from build123d import *

# Parameters (mm, degrees)
F0_W           = 60
F0_H           = 35
F1_DEPTH       = 4
F3_DEPTH       = 3
F4_R           = 5.08
F5_W           = 27
F5_H           = 19
F6_DEPTH       = 25.4
F8_D           = 3.5
F8_CSINK_D     = 6
F8_CSINK_ANGLE = 90
F9_D           = 3
F10_T1_DEPTH   = 58
F10_T3_DEPTH   = 33
F10_T5_DEPTH   = 5.5
F10_S9_W       = 1
F10_S9_H       = 1
F10_T10_DEPTH  = 1
F10_S15_W      = 1
F10_S15_H      = 1
F10_T16_DEPTH  = 1
F10_S21_W      = 1
F10_S21_H      = 1
F10_T22_DEPTH  = 1
F10_S27_W      = 1
F10_S27_H      = 1
F10_T28_DEPTH  = 1


# Not quite as in the source:
# - a fillet or chamfer that OpenCascade refuses, or shapes differently, is made with other operations: its cross-section is extruded or revolved along the edge and cut away or added


with BuildPart() as f1:
    # F0 (on Top) → F1 (new body)
    with BuildSketch(Plane.XY):
        Rectangle(F0_W, F0_H)
    extrude(amount=F1_DEPTH)

    # F2 (on face) → F3 (cut)
    with BuildSketch(Plane.XY.offset(4)):
        Polygon((-27.3, 0), (-12.5, -11.5), (12.5, -11.5), (27.3, 0), (12.5, 11.5), (-12.5, 11.5), align=None)
    extrude(amount=-F3_DEPTH, mode=Mode.SUBTRACT)

    # F4
    f4_edges = [f1.edges().sort_by_distance(p)[0] for p in [
        (12.5, 11.5, 2.5),
        (12.5, -11.5, 2.5),
        (-12.5, -11.5, 2.5),
        (-12.5, 11.5, 2.5),
        (27.3, 0, 2.5),
        (-27.3, 0, 2.5),
    ]]
    fillet(f4_edges, radius=F4_R)

    # F5 (on face) → F6 (cut)
    with BuildSketch(Plane.XY.offset(1)):
        Rectangle(F5_W, F5_H)
    extrude(amount=-F6_DEPTH, mode=Mode.SUBTRACT)

    # F8 (through all)
    with Locations(Plane.XY.offset(4)):
        with Locations((-26, 13.5), (26, 13.5), (26, -13.5), (-26, -13.5)):
            CounterSinkHole(F8_D / 2, F8_CSINK_D / 2, counter_sink_angle=F8_CSINK_ANGLE)

    # F9 (through all)
    with Locations(Plane.XY.offset(4)):
        with Locations((-20.3, 0), (20.3, 0)):
            Hole(F9_D / 2)

    # F10: fillet of radius 1 on 8 edges, made by hand

    # F10_s2 → F10_t1 (cut)
    with BuildSketch(Plane.YZ.offset(-29)):
        with BuildLine():
            ThreePointArc((16.5, 4), (17.2071067812, 3.7071067812), (17.5, 3))
            Line((17.5, 3), (17.5, 4))
            Line((17.5, 4), (16.5, 4))
        make_face()
        with BuildLine():
            ThreePointArc((-16.5, 4), (-17.2071067812, 3.7071067812), (-17.5, 3))
            Line((-17.5, 3), (-17.5, 4))
            Line((-17.5, 4), (-16.5, 4))
        make_face()
    extrude(amount=F10_T1_DEPTH, mode=Mode.SUBTRACT)

    # F10_s4 → F10_t3 (cut)
    with BuildSketch(Plane.XZ.offset(-16.5)):
        with BuildLine():
            ThreePointArc((-29, 4), (-29.7071067812, 3.7071067812), (-30, 3))
            Line((-30, 3), (-30, 4))
            Line((-30, 4), (-29, 4))
        make_face()
        with BuildLine():
            ThreePointArc((29, 4), (29.7071067812, 3.7071067812), (30, 3))
            Line((30, 3), (30, 4))
            Line((30, 4), (29, 4))
        make_face()
    extrude(amount=F10_T3_DEPTH, mode=Mode.SUBTRACT)

    # F10_s6 → F10_t5 (cut)
    with BuildSketch(Plane.XY.offset(-2.5)):
        with BuildLine():
            ThreePointArc((30, -16.5), (29.7071067812, -17.2071067812), (29, -17.5))
            Line((29, -17.5), (30, -17.5))
            Line((30, -17.5), (30, -16.5))
        make_face()
        with BuildLine():
            ThreePointArc((29, 17.5), (29.7071067812, 17.2071067812), (30, 16.5))
            Line((30, 16.5), (30, 17.5))
            Line((30, 17.5), (29, 17.5))
        make_face()
        with BuildLine():
            ThreePointArc((-30, -16.5), (-29.7071067812, -17.2071067812), (-29, -17.5))
            Line((-29, -17.5), (-30, -17.5))
            Line((-30, -17.5), (-30, -16.5))
        make_face()
        with BuildLine():
            ThreePointArc((-29, 17.5), (-29.7071067812, 17.2071067812), (-30, 16.5))
            Line((-30, 16.5), (-30, 17.5))
            Line((-30, 17.5), (-29, 17.5))
        make_face()
    extrude(amount=F10_T5_DEPTH, mode=Mode.SUBTRACT)


with BuildPart() as f10_tool8:
    # F10_s9 → F10_t10 (new body)
    with BuildSketch(Plane.XY.offset(3)):
        with Locations((29.5, 17)):
            Rectangle(F10_S9_W, F10_S9_H)
    extrude(amount=F10_T10_DEPTH)

    # F10_s11 → F10_t12 (revolve, cut)
    with BuildSketch(Plane(origin=(29, 16.5, 3), x_dir=(-0.7071067812, -0.7071067812, 0), z_dir=(-0.7071067812, 0.7071067812, 0))):
        with BuildLine():
            ThreePointArc((0, -1), (1, 0), (0, 1))
            Line((0, 1), (0, -1))
        make_face()
    revolve(axis=Axis((29, 16.5, 3), (0, 0, 1)), mode=Mode.SUBTRACT)


with BuildPart() as f1_1:
    add(f1.part)

    # F10_t7: cut F10_tool8
    add(f10_tool8.part, mode=Mode.SUBTRACT)


with BuildPart() as f10_tool14:
    # F10_s15 → F10_t16 (new body)
    with BuildSketch(Plane.XY.offset(3)):
        with Locations((-29.5, 17)):
            Rectangle(F10_S15_W, F10_S15_H)
    extrude(amount=F10_T16_DEPTH)

    # F10_s17 → F10_t18 (revolve, cut)
    with BuildSketch(Plane(origin=(-29, 16.5, 3), x_dir=(0.7071067812, -0.7071067812, 0), z_dir=(-0.7071067812, -0.7071067812, 0))):
        with BuildLine():
            ThreePointArc((0, -1), (1, 0), (0, 1))
            Line((0, 1), (0, -1))
        make_face()
    revolve(axis=Axis((-29, 16.5, 3), (0, 0, 1)), mode=Mode.SUBTRACT)


with BuildPart() as f1_2:
    add(f1_1.part)

    # F10_t13: cut F10_tool14
    add(f10_tool14.part, mode=Mode.SUBTRACT)


with BuildPart() as f10_tool20:
    # F10_s21 → F10_t22 (new body)
    with BuildSketch(Plane.XY.offset(3)):
        with Locations((-29.5, -17)):
            Rectangle(F10_S21_W, F10_S21_H)
    extrude(amount=F10_T22_DEPTH)

    # F10_s23 → F10_t24 (revolve, cut)
    with BuildSketch(Plane(origin=(-29, -16.5, 3), x_dir=(0.7071067812, 0.7071067812, 0), z_dir=(0.7071067812, -0.7071067812, 0))):
        with BuildLine():
            ThreePointArc((0, -1), (1, 0), (0, 1))
            Line((0, 1), (0, -1))
        make_face()
    revolve(axis=Axis((-29, -16.5, 3), (0, 0, 1)), mode=Mode.SUBTRACT)


with BuildPart() as f1_3:
    add(f1_2.part)

    # F10_t19: cut F10_tool20
    add(f10_tool20.part, mode=Mode.SUBTRACT)


with BuildPart() as f10_tool26:
    # F10_s27 → F10_t28 (new body)
    with BuildSketch(Plane.XY.offset(3)):
        with Locations((29.5, -17)):
            Rectangle(F10_S27_W, F10_S27_H)
    extrude(amount=F10_T28_DEPTH)

    # F10_s29 → F10_t30 (revolve, cut)
    with BuildSketch(Plane(origin=(29, -16.5, 3), x_dir=(-0.7071067812, 0.7071067812, 0), z_dir=(0.7071067812, 0.7071067812, 0))):
        with BuildLine():
            ThreePointArc((0, -1), (1, 0), (0, 1))
            Line((0, 1), (0, -1))
        make_face()
    revolve(axis=Axis((29, -16.5, 3), (0, 0, 1)), mode=Mode.SUBTRACT)


with BuildPart() as f1_4:
    add(f1_3.part)

    # F10_t25: cut F10_tool26
    add(f10_tool26.part, mode=Mode.SUBTRACT)


solid = f1_4.part
Verification items for the finished model (mm, model axes). A direction names the side the tool comes from. Round coordinates to 2 decimals unless told otherwise and drop trailing zeros. Loops run counter-clockwise (first coordinate to the right, second up) from the corner with the lowest first, then second, coordinate; pieces in that order, holes last. Notation, with made-up numbers: (7.25, -22) - (13.25, -22) arc R29 ccw to (13.25, -1) - close; hole circle Ø7 at (87, 30). An arc over 180 degrees is marked (long way). Answer in a Markdown table with one row per item. Add a question column.
Q1. Release check for a two-part mould opening along Y. For faces 1 (the face through (0, 17.5, 1)), 2 (the face through (0, 15, 4)), 3 (the face through (2, 10, 1)) record: pulls with the +Y half, pulls with the -Y half, needs draft (parallel to the pull), parting line crosses it, or undercut.
Q2. Section check B-B on y = 0. Enter the section's corners in (x, z), plus the area to 3 significant figures.
Q3. Material ranges on line 1 (Y direction, x = 26, z = 1.65); line 2 (Y direction, x = 2, z = 1.8); line 3 (Y direction, x = -3.5, z = 0.8), recorded low to high.
Q4. Tool access check on faces 4 (the face through (18.06, 7.18, 2.52)), 5 (the face through (21.8, 0.07, 0.49)). Record the directions out of +Z, -Z, +X, -X, +Y, -Y that give a thin tool (end or side, any length) a straight path to the whole face; none if there is none.
Q5. Section check A-A on z = 1.85. Enter the section's corners in (x, y), plus the area to 3 significant figures.
Q6. Section check C-C on x = -20.3. Enter the section's corners in (y, z).
Q7. Gauge pin test, flat end, axial feed: pin 1 (12 mm diameter, centred on x = -10.5, y = -2.5, fed in from +Z). Record the tip position at first contact, or that the pin passes through.
Found:
| question | item | result |
|---|---|---|
| 1 | face 1 | pulls with the +Y half |
| 1 | face 2 | needs draft |
| 1 | face 3 | undercut |
| 2 | outline | (-30, 0) - (-21.8, 0) - (-21.8, 1) - (-24.1, 1) - (-24.1, 4) - (-29, 4) arc R1 ccw to (-30, 3) - close; (-18.8, 0) - (-13.5, 0) - (-13.5, 1) - (-18.8, 1) - close; (13.5, 0) - (18.8, 0) - (18.8, 1) - (13.5, 1) - close; (21.8, 0) - (30, 0) - (30, 3) arc R1 ccw to (29, 4) - (24.1, 4) - (24.1, 1) - (21.8, 1) - close |
| 2 | area | 62.0 mm² |
| 3 | line 1 | y = -17.5 to -15.25, -11.75 to 11.75, 15.25 to 17.5 |
| 3 | line 2 | y = -17.5 to -11.5, 11.5 to 17.5 |
| 3 | line 3 | y = -17.5 to -9.5, 9.5 to 17.5 |
| 4 | face 4 | +Z |
| 4 | face 5 | +Z, -Z |
| 5 | outline | (-30, -16.5) arc R1 ccw to (-29, -17.5) - (29, -17.5) arc R1 ccw to (30, -16.5) - (30, 16.5) arc R1 ccw to (29, 17.5) - (-29, 17.5) arc R1 ccw to (-30, 16.5) - close; hole circle Ø3.5 at (-26, -13.5); hole circle Ø3.5 at (-26, 13.5); hole (-22.14, -4.01) - (-13.88, -10.43) arc R5.08 ccw to (-10.76, -11.5) - (10.76, -11.5) arc R5.08 ccw to (13.88, -10.43) - (22.14, -4.01) arc R5.08 ccw to (22.14, 4.01) - (13.88, 10.43) arc R5.08 ccw to (10.76, 11.5) - (-10.76, 11.5) arc R5.08 ccw to (-13.88, 10.43) - (-22.14, 4.01) arc R5.08 ccw to start; hole circle Ø3.5 at (26, -13.5); hole circle Ø3.5 at (26, 13.5) |
| 5 | area | 1,170 mm² |
| 6 | outline | (-17.5, 0) - (-1.5, 0) - (-1.5, 1) - (-5.44, 1) - (-5.44, 4) - (-16.5, 4) arc R1 ccw to (-17.5, 3) - close; (1.5, 0) - (17.5, 0) - (17.5, 3) arc R1 ccw to (16.5, 4) - (5.44, 4) - (5.44, 1) - (1.5, 1) - close |
| 7 | pin 1 | stops at z = 1 |
